```python
from build123d import *

# Parameters (mm, degrees)
SKETCH_1_R               = 150
EXTRUDE_1_DEPTH          = 4
SKETCH_2_R               = 150
SKETCH_2_R_2             = 145.8
EXTRUDE_2_DEPTH          = 50
SKETCH_3_R               = 145.8
SKETCH_3_R_2             = 142.8
EXTRUDE_3_DEPTH          = 62
CUT_EXTRUDE_1_DEPTH      = 223.162102979
CUT_EXTRUDE_1_DEPTH_BACK = 223.162102979
EXTRUDE_4_DEPTH          = 50
CUT_EXTRUDE_START        = -12
CUT_EXTRUDE_2_DEPTH      = 12
FILLET_1_R               = 5
CUT_EXTRUDE_3_DEPTH      = 223.162103114
CUT_EXTRUDE_3_DEPTH_BACK = 223.162103114
SKETCH_7_R               = 35
CUT_EXTRUDE_4_DEPTH      = 25
SKETCH_9_W               = 10
SKETCH_9_H               = 20
CUT_EXTRUDE_5_DEPTH      = 25
SKETCH_10_R              = 17.2
CUT_EXTRUDE_6_DEPTH      = 25
EXTRUDE_START            = 4
EXTRUDE_5_DEPTH          = 4
SKETCH_12_R              = 5
SKETCH_12_R_2            = 2
SKETCH_12_R_3            = 5.00000108
SKETCH_12_R_4            = 2.00000108
EXTRUDE_6_DEPTH          = 5
CHAMFER_1_SIZE           = 2
CHAMFER_2_SIZE           = 3
SKETCH_13_W              = 15
SKETCH_13_H              = 30
CUT_EXTRUDE_7_DEPTH      = 223.162103114


with BuildPart() as part:
    # 스케치1 → 보스-돌출1 (new body)
    with BuildSketch(Plane(origin=(0, 0, 0), x_dir=(1, 0, 0), z_dir=(0, 1, 0))):
        with Locations(Location((0, 0, 0), (0, 0, 270))):
            Circle(SKETCH_1_R)
    extrude(amount=EXTRUDE_1_DEPTH)

    # 스케치2 → 보스-돌출2 (add)
    with BuildSketch(Plane(origin=(0, 4, 0), x_dir=(1, 0, 0), z_dir=(0, 1, 0))):
        with Locations(Location((0, 0, 0), (0, 0, 270))):
            Circle(SKETCH_2_R)
        with Locations(Location((0, 0, 0), (0, 0, 270))):
            Circle(SKETCH_2_R_2, mode=Mode.SUBTRACT)
    extrude(amount=EXTRUDE_2_DEPTH)

    # 스케치3 → 보스-돌출3 (add)
    with BuildSketch(Plane(origin=(0, 4, 0), x_dir=(1, 0, 0), z_dir=(0, 1, 0))):
        with Locations(Location((0, 0, 0), (0, 0, 270))):
            Circle(SKETCH_3_R)
        with Locations(Location((0, 0, 0), (0, 0, 270))):
            Circle(SKETCH_3_R_2, mode=Mode.SUBTRACT)
    extrude(amount=EXTRUDE_3_DEPTH)

    # 스케치4 → 컷-돌출1 (cut, two sides: drawn at the far end of the back side and taken through both)
    with BuildSketch(Plane.XZ.offset(-CUT_EXTRUDE_1_DEPTH_BACK)):
        with BuildLine():
            Line((85.8, 73), (85.8, 123.038042897))
            ThreePointArc((85.8, 123.038042897), (0, 150), (-85.8, 123.038042897))
            Line((-85.8, 123.038042897), (-85.8, 73))
            Line((-85.8, 73), (-84.8, 72))
            Line((-84.8, 72), (84.8, 72))
            Line((84.8, 72), (85.8, 73))
        make_face()
    extrude(amount=CUT_EXTRUDE_1_DEPTH + CUT_EXTRUDE_1_DEPTH_BACK, mode=Mode.SUBTRACT)

    # 스케치5 → 보스-돌출4 (add)
    with BuildSketch(Plane(origin=(0, 4, 0), x_dir=(1, 0, 0), z_dir=(0, 1, 0))):
        with BuildLine():
            Line((-86.456854249, -68), (-89.8, -71.343145751))
            Line((-89.8, -71.343145751), (-89.8, -114.149901445))
            Line((-89.8, -114.149901445), (-89.8, -114.863397129))
            ThreePointArc((-89.8, -114.863397129), (-87.812965607, -116.389531622), (-85.8, -117.881296226))
            Line((-85.8, -117.881296226), (-85.8, -72))
            Line((-85.8, -72), (85.8, -72))
            Line((85.8, -72), (85.8, -117.881296226))
            ThreePointArc((85.8, -117.881296226), (87.812965607, -116.389531622), (89.8, -114.863397129))
            Line((89.8, -114.863397129), (89.8, -114.149901445))
            Line((89.8, -114.149901445), (89.8, -71.343145751))
            Line((89.8, -71.343145751), (86.45685425, -68))
            Line((86.45685425, -68), (84.8, -68))
            Line((84.8, -68), (-84.8, -68))
            Line((-84.8, -68), (-86.456854249, -68))
        make_face()
        Polygon((-89.8, -68), (-89.8, -71.343145751), (-86.456854249, -68), align=None)
        Polygon((89.8, -68), (86.45685425, -68), (89.8, -71.343145751), align=None)
    extrude(amount=EXTRUDE_4_DEPTH)

    # 스케치6 → 컷-돌출2 (cut)
    with BuildSketch(Plane(origin=(0, 66, 0), x_dir=(1, 0, 0), z_dir=(0, 1, 0)).offset(CUT_EXTRUDE_START)):
        with BuildLine():
            Line((-89.8, -114.149901445), (-89.674405594, -111.132087991))
            ThreePointArc((-89.674405594, -111.132087991), (-87.750176947, -112.657651519), (-85.8, -114.149901445))
            Line((-85.8, -114.149901445), (-85.8, -117.881296226))
            ThreePointArc((-85.8, -117.881296226), (-87.812965607, -116.389531622), (-89.8, -114.863397129))
            Line((-89.8, -114.863397129), (-89.8, -114.149901445))
        make_face()
    cut_extrude_2 = extrude(amount=CUT_EXTRUDE_2_DEPTH, mode=Mode.SUBTRACT)

    # 대칭 복사1: 컷-돌출2 across plane
    add(cut_extrude_2.mirror(Plane(origin=(0, 0, 0), x_dir=(0, 0, 1), z_dir=(1, 0, 0))), mode=Mode.SUBTRACT)

    # 필렛1
    fillet_1_edges = [part.edges().sort_by_distance(p)[0] for p in [
        (0, 0, -150),
    ]]
    fillet(fillet_1_edges, radius=FILLET_1_R)

    # 스케치7 → 컷-돌출3 (cut, two sides: drawn at the far end of the back side and taken through both)
    with BuildSketch(Plane.XZ.offset(-CUT_EXTRUDE_3_DEPTH_BACK)):
        with Locations(Location((0, 0, 0), (0, 0, 90))):
            Circle(SKETCH_7_R)
    extrude(amount=CUT_EXTRUDE_3_DEPTH + CUT_EXTRUDE_3_DEPTH_BACK, mode=Mode.SUBTRACT)

    # 스케치8 → 컷-돌출4 (cut)
    with BuildSketch(Plane(origin=(0, 54, 0), x_dir=(1, 0, 0), z_dir=(0, 1, 0))):
        with BuildLine():
            ThreePointArc((0, 150), (-15.67926949, 149.178284305), (-31.186753623, 146.72214011))
            Line((-31.186753623, 146.72214011), (-30.313524521, 142.613920187))
            ThreePointArc((-30.313524521, 142.613920187), (-15.240249944, 145.001292345), (0, 145.8))
            Line((0, 145.8), (0, 150))
        make_face()
        with BuildLine():
            ThreePointArc((0, 145.8), (-15.240249944, 145.001292345), (-30.313524521, 142.613920187))
            Line((-30.313524521, 142.613920187), (-29.523460096, 138.896959304))
            ThreePointArc((-29.523460096, 138.896959304), (-14.843041784, 141.222109142), (0, 142))
            Line((0, 142), (0, 145.8))
        make_face()
        with BuildLine():
            ThreePointArc((-90.633052966, 108.01226648), (-118.91819386, 75.759244777), (-136.195541507, 36.493485359))
            Line((-136.195541507, 36.493485359), (-140.059244812, 37.52876154))
            Line((-140.059244812, 37.52876154), (-144.888873943, 38.822856765))
            ThreePointArc((-144.888873943, 38.822856765), (-126.508716872, 80.594941252), (-96.418141453, 114.906666468))
            Line((-96.418141453, 114.906666468), (-93.204203405, 111.076444252))
            Line((-93.204203405, 111.076444252), (-90.633052966, 108.01226648))
        make_face()
    cut_extrude_4 = extrude(amount=CUT_EXTRUDE_4_DEPTH, mode=Mode.SUBTRACT)

    # 대칭 복사2: 컷-돌출4 across plane
    add(cut_extrude_4.mirror(Plane(origin=(0, 0, 0), x_dir=(0, 0, 1), z_dir=(1, 0, 0))), mode=Mode.SUBTRACT)

    # 스케치9 → 컷-돌출5 (cut)
    with BuildSketch(Plane.XZ):
        with Locations((0, -35)):
            Rectangle(SKETCH_9_W, SKETCH_9_H)
    extrude(amount=-CUT_EXTRUDE_5_DEPTH, mode=Mode.SUBTRACT)

    # 스케치10 → 컷-돌출6 (cut)
    with BuildSketch(Plane(origin=(0, 0, 68), x_dir=(-1, 0, 0), z_dir=(0, 0, -1))):
        with Locations((0.117103381, 49)):
            Circle(SKETCH_10_R)
    extrude(amount=-CUT_EXTRUDE_6_DEPTH, mode=Mode.SUBTRACT)

    # 스케치11 → 보스-돌출5 (add)
    with BuildSketch(Plane(origin=(0, 0, 68), x_dir=(-1, 0, 0), z_dir=(0, 0, -1)).offset(EXTRUDE_START)):
        with BuildLine():
            Line((17.317103381, 49), (21.317103381, 49))
            ThreePointArc((21.317103381, 49), (0.117103381, 27.8), (-21.082896619, 49))
            Line((-21.082896619, 49), (-17.082896619, 49))
            ThreePointArc((-17.082896619, 49), (0.117103381, 31.8), (17.317103381, 49))
        make_face()
    extrude(amount=-EXTRUDE_5_DEPTH)

    # 스케치12 → 보스-돌출6 (add)
    # profile 1 of 6: a face of its own
    with BuildSketch(Plane(origin=(0, 4, 0), x_dir=(1, 0, 0), z_dir=(0, 1, 0))):
        with Locations(Location((100, 35, 0), (0, 0, 270))):
            Circle(SKETCH_12_R)
        with Locations(Location((100, 35, 0), (0, 0, 270))):
            Circle(SKETCH_12_R_2, mode=Mode.SUBTRACT)
    # profile 2 of 6: a face of its own
    with BuildSketch(Plane(origin=(0, 4, 0), x_dir=(1, 0, 0), z_dir=(0, 1, 0))):
        with Locations(Location((-100, 35, 0), (0, 0, 270))):
            Circle(SKETCH_12_R)
        with Locations(Location((-100, 35, 0), (0, 0, 270))):
            Circle(SKETCH_12_R_2, mode=Mode.SUBTRACT)
    # profile 3 of 6: a face of its own
    with BuildSketch(Plane(origin=(0, 4, 0), x_dir=(1, 0, 0), z_dir=(0, 1, 0))):
        with Locations(Location((-79.999996057, 83.000003885, 0), (0, 0, 270))):
            Circle(SKETCH_12_R_3)
        with Locations(Location((-79.999996057, 83.000003885, 0), (0, 0, 270))):
            Circle(SKETCH_12_R_4, mode=Mode.SUBTRACT)
    # profile 4 of 6: a face of its own
    with BuildSketch(Plane(origin=(0, 4, 0), x_dir=(1, 0, 0), z_dir=(0, 1, 0))):
        with Locations(Location((-29.99999481, 120.000031962, 0), (0, 0, 270))):
            Circle(SKETCH_12_R_3)
        with Locations(Location((-29.99999481, 120.000031962, 0), (0, 0, 270))):
            Circle(SKETCH_12_R_4, mode=Mode.SUBTRACT)
    # profile 5 of 6: a face of its own
    with BuildSketch(Plane(origin=(0, 4, 0), x_dir=(1, 0, 0), z_dir=(0, 1, 0))):
        with Locations(Location((29.99998679, 120.000032533, 0), (0, 0, 270))):
            Circle(SKETCH_12_R_3)
        with Locations(Location((29.99998679, 120.000032533, 0), (0, 0, 270))):
            Circle(SKETCH_12_R_4, mode=Mode.SUBTRACT)
    # profile 6 of 6: a face of its own
    with BuildSketch(Plane(origin=(0, 4, 0), x_dir=(1, 0, 0), z_dir=(0, 1, 0))):
        with Locations(Location((79.999988743, 83.000005409, 0), (0, 0, 270))):
            Circle(SKETCH_12_R_3)
        with Locations(Location((79.999988743, 83.000005409, 0), (0, 0, 270))):
            Circle(SKETCH_12_R_4, mode=Mode.SUBTRACT)
    extrude(amount=EXTRUDE_6_DEPTH)

    # 모따기1
    chamfer_1_edges = [part.edges().sort_by_distance(p)[0] for p in [
        (100, 4, -40),
        (-79.999996057, 4, -88.000004965),
        (-100, 4, -40),
        (-29.99999481, 4, -125.000033042),
        (29.99998679, 4, -125.000033613),
        (79.999988743, 4, -88.000006489),
    ]]
    chamfer(chamfer_1_edges, length=CHAMFER_1_SIZE)

    # 모따기2
    chamfer_2_edges = [part.edges().sort_by_distance(p)[0] for p in [
        (0, 0, 72),
    ]]
    chamfer(chamfer_2_edges, length=CHAMFER_2_SIZE)

    # 스케치13 → 컷-돌출7 (cut, through all)
    with BuildSketch(Plane.XY):
        with Locations((-40, 30)):
            Rectangle(SKETCH_13_W, SKETCH_13_H)
        with Locations((40, 30)):
            Rectangle(SKETCH_13_W, SKETCH_13_H)
    extrude(amount=-CUT_EXTRUDE_7_DEPTH, mode=Mode.SUBTRACT)


solid = part.part
```
Check sheet for the modelled part. Datum: model origin and axes. Units: mm. A direction names the side the tool comes from. Coordinates: 2 decimals unless noted, no trailing zeros. Order: outer loops, then holes, each group sorted by start corner. A loop starts at its lowest first (then second) coordinate and runs counter-clockwise, first axis right, second up. Notation, with made-up numbers: (-33.75, 28.5) -> (17.25, 28.5) arc R23 cw to (17.25, 40.5) -> close; hole circle Ø9 at (34, -17.75). An arc over 180 degrees is marked (long way). Write each question's results on one line, items separated by ' | '. Start each with the question number.
1) Draft check along Y on faces 5 (the face through (47.5, 30, -138)), 6 (the face through (78.085, 7.479, -78.381)), 7 (the face through (34, 0, -16)). Enter one of: pulls with the +Y half, pulls with the -Y half, needs draft (parallel to the pull), parting line crosses it, or undercut.
2) Section check B-B (y = 61.5). Enter the section's corners in (x, z).
3) Section check A-A (z = 0). Enter the section's corners in (x, y), and give its area (3 significant figures).
4) Set-up check for faces 1 (the face through (-63.47, 59.92, -131.26)), 2 (the face through (-138.647, 59.916, 45.108)), 3 (the face through (0, 31, 64)), 4 (the face through (-47.5, 30, -138)): record each of +Z, -Z, +X, -X, +Y, -Y from which the full face is reachable in a straight line by a thin tool's end or side.
5) Material ranges on line 1 along X through (y, z) = (48.5, 0); line 2 along X through (y, z) = (6.2, -35); line 3 along Z through (x, y) = (84.5, 8.5), recorded low to high.
6) Depth check by flat-ended pin: pin 1 (1.2 mm diameter, centred on x = 18.5, z = 67, fed in from +Y); pin 2 (2 mm diameter, centred on y = 1.5, z = -39, fed in from -X); pin 3 (12 mm diameter, centred on x = -33, z = 40.5, fed in from +Y); pin 4 (2.5 mm diameter, centred on x = -30, z = -120, fed in from -Y). Enter the tip coordinate at first touch or a pass-through.
Checked values:
1) face 5: undercut | face 6: needs draft | face 7: pulls with the -Y half
2) outline: (-140.83, -37.74) -> (-137.93, -36.96) arc R142.8 cw to (-89.67, 111.13) -> (-89.8, 114.15) -> (-89.8, 114.86) arc R145.8 ccw to start; (-93.72, -111.69) arc R145.8 ccw to (-30.31, -142.61) -> (-29.69, -139.68) arc R142.8 cw to (-91.79, -109.39) -> close; (29.69, -139.68) -> (30.31, -142.61) arc R145.8 ccw to (93.72, -111.69) -> (91.79, -109.39) arc R142.8 cw to start; (89.67, 111.13) arc R142.8 cw to (137.93, -36.96) -> (140.83, -37.74) arc R145.8 ccw to (89.8, 114.86) -> (89.8, 114.15) -> close
3) outline: (-150, 5) arc R5 ccw to (-145, 0) -> (-35, 0) -> (-35, 4) -> (-142.8, 4) -> (-142.8, 66) -> (-145.8, 66) -> (-145.8, 54) -> (-150, 54) -> close; (35, 0) -> (145, 0) arc R5 ccw to (150, 5) -> (150, 54) -> (145.8, 54) -> (145.8, 66) -> (142.8, 66) -> (142.8, 4) -> (35, 4) -> close | area: 1,700 mm²
4) face 1: -Z, -X, +Y | face 2: -X, +Y | face 3: +Y | face 4: -Z
5) line 1: -150 to -142.8, 142.8 to 150 | line 2: -145.86 to -138.44, -105 to -102, -98 to -95, 95 to 98, 102 to 105, 138.44 to 145.86 | line 3: -123.93 to -115.12, -85.18 to -80.82, 68 to 72
6) pin 1: y = 49 | pin 2: x = -144.2 | pin 3: y = 4 | pin 4: y = 0
